```python
from build123d import *

# Parameters (mm, degrees)
F0_R     = 9.525
F1_DEPTH = 19.05


with BuildPart() as f1:
    # F0 (on Front) → F1 (new body)
    with BuildSketch(Plane.XZ):
        with BuildLine():
            ThreePointArc((14.2875, 12.600391), (-12.600391, 14.2875), (-14.2875, -12.600391))
            ThreePointArc((-14.2875, -12.600391), (95.25, -62.047396), (204.7875, -12.600391))
            ThreePointArc((204.7875, -12.600391), (203.100391, 14.2875), (176.2125, 12.600391))
            ThreePointArc((176.2125, 12.600391), (95.25, -23.947396), (14.2875, 12.600391))
        make_face()
        Circle(F0_R, mode=Mode.SUBTRACT)
        with Locations((190.5, 0)):
            Circle(F0_R, mode=Mode.SUBTRACT)
    extrude(amount=F1_DEPTH)


solid = f1.part
```
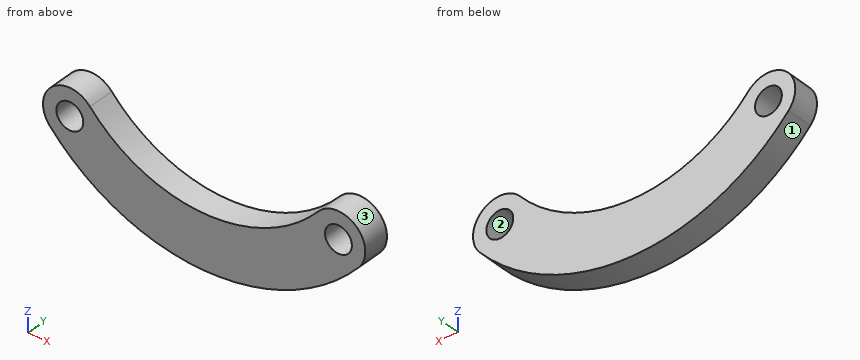
CAD build for the part. Positions are in the model's coordinates, mm. Face numbers are marked on the shaded views. Round coordinates to 2 decimals unless told otherwise and drop trailing zeros. Order: outer loops, then holes, each group sorted by start corner. A loop starts at its lowest first (then second) coordinate and runs counter-clockwise, first axis right, second up.
Q1. Two-plate mould, pull along Z, no slides. Class the marked faces 1, 2 and 3: pulls with the +Z half, pulls with the -Z half, needs draft (parallel to the pull), parting line crosses it, or undercut.
Q2. Wall check: L1, parallel to X at y = -13.5, z = -4.5; L2, parallel to Z at x = 190.5, y = -5.5 (3 decimals); L3, parallel to X at y = -13, z = 0.5. Give the ranges that are in metal, low to high.
Q3. Drop flat-ended pins along their axis: pin 1 (2 mm diameter, centred on x = 183, y = -5.5, fed in from -Z); pin 2 (1 mm diameter, centred on y = -4.5, z = -19, fed in from +X); pin 3 (1.5 mm diameter, centred on y = -9, z = -44, fed in from +X); pin 4 (15 mm diameter, centred on x = 0, z = 0, fed in from +Y). Give the stop position or say it passes through.
Q4. Slice it at C-C (y = -11.25). State how many separate pieces and enclosed holes the cut face has, and give its area (3 significant figures).
Q5. Slice it at B-B (z = -20.5). Write the cut outline in (x, y), and give its area (3 significant figures).
Q6. Slice it at A-A (x = 190.5). Write the cut outline in (y, z) (3 decimals).
Q7. Slice it at D-D (z = 0). Write the cut outline in (x, y) (3 decimals), and give its area (3 significant figures).
Results below:
1. face 1: pulls with the -Z half
1. face 2: undercut
1. face 3: parting line crosses it
2. L1: x = -18.51 to -8.39, 8.39 to 33.44, 157.06 to 182.11, 198.89 to 209.01
2. L2: z = -26.713 to -9.525, 9.525 to 19.05
2. L3: x = -19.04 to -9.51, 9.51 to 26.84, 163.66 to 180.99, 200.01 to 209.54
3. pin 1: stops at z = -33.49
3. pin 2: stops at x = 199.29
3. pin 3: stops at x = 166.93
3. pin 4: passes through
4. separate pieces: 1
4. enclosed holes: 2
4. area: 8,780 mm2
5. outline: (-6.78, -19.05) - (68.19, -19.05) - (68.19, 0) - (-6.78, 0) - close; (122.31, -19.05) - (197.28, -19.05) - (197.28, 0) - (122.31, 0) - close
5. area: 2,860 mm2
6. outline: (-19.05, -26.713) - (0, -26.713) - (0, -9.525) - (-19.05, -9.525) - close; (-19.05, 9.525) - (0, 9.525) - (0, 19.05) - (-19.05, 19.05) - close
7. outline: (-19.05, -19.05) - (-9.525, -19.05) - (-9.525, 0) - (-19.05, 0) - close; (9.525, -19.05) - (27.451, -19.05) - (27.451, 0) - (9.525, 0) - close; (163.049, -19.05) - (180.975, -19.05) - (180.975, 0) - (163.049, 0) - close; (200.025, -19.05) - (209.55, -19.05) - (209.55, 0) - (200.025, 0) - close
7. area: 1,050 mm2
